```python
from build123d import *

# Parameters (mm, degrees)
PAD_DEPTH       = 15
FILLET_R        = 10
FILLET001_R     = 3
CHAMFER_SIZE    = 2
FILLET002_R     = 0.5
FILLET003_R     = 5
CHAMFER001_SIZE = 0.25
SKETCH003_R     = 1.5
POCKET_DEPTH    = 33.001


with BuildPart() as sweep_body:
    # Sweep: sweep along a path in Sketch001
    with BuildLine(Plane.XY) as sweep_path:
        Line((21, -10), (21, 15.000008))
        ThreePointArc((21, 15.000008), (18.071065, 22.071071), (11, 25))
        Line((11, 25), (-11, 25))
        ThreePointArc((-11, 25), (-18.071068, 22.071068), (-21, 15))
        Line((-21, 15), (-21, -10))
    # Sketch002 → Sweep (sweep)
    with BuildSketch(Plane.XZ.offset(10)):
        Polygon((22, 3.25), (22, -3.25), (20, -1.25), (20, 1.25), align=None)
    sweep(path=sweep_path.line)


with BuildPart() as sweep_body_1:
    # Sweep placement: moved
    add(sweep_body.part.moved(Location((0, 0, 3))))


with BuildPart() as fusion:
    # Clone base: copy of Sweep body
    add(sweep_body_1.part)


with BuildPart() as fusion_1:
    # Clone placement: moved
    add(fusion.part.moved(Location((0, 0, 9))))

    # Fusion: union Sweep body
    add(sweep_body_1.part)


with BuildPart() as pocket:
    # Sketch → Pad (new body)
    with BuildSketch(Plane.XY):
        Polygon((-18, -8), (-18, 12), (-12, 18), (12, 18), (18, 12), (18, -8), (21, -8), (21, 25), (-21, 25), (-21, -8), align=None)
    extrude(amount=PAD_DEPTH)

    # Fillet
    fillet_edges = [pocket.edges().sort_by_distance(p)[0] for p in [
        (-21, 25, 7.5),
        (21, 25, 7.5),
    ]]
    fillet(fillet_edges, radius=FILLET_R)

    # Fillet001
    fillet001_edges = [pocket.edges().sort_by_distance(p)[0] for p in [
        (-12, 18, 7.5),
        (-18, 12, 7.5),
        (12, 18, 7.5),
        (18, 12, 7.5),
    ]]
    fillet(fillet001_edges, radius=FILLET001_R)

    # Chamfer
    chamfer_edges = [pocket.edges().sort_by_distance(p)[0] for p in [
        (-21, -8, 7.5),
        (21, -8, 7.5),
    ]]
    chamfer(chamfer_edges, length=CHAMFER_SIZE)

    # Fillet002
    fillet002_edges = [pocket.edges().sort_by_distance(p)[0] for p in [
        (-19, -8, 7.5),
        (-18, -8, 7.5),
        (19, -8, 7.5),
        (18, -8, 7.5),
    ]]
    fillet(fillet002_edges, radius=FILLET002_R)

    # Fillet003
    fillet003_edges = [pocket.edges().sort_by_distance(p)[0] for p in [
        (-21, -6, 7.5),
        (21, -6, 7.5),
    ]]
    fillet(fillet003_edges, radius=FILLET003_R)

    # Chamfer001
    chamfer001_edges = [pocket.edges().sort_by_distance(p)[0] for p in [
        (19.34099, -7.65901, 15),
        (20.619398, -5.842349, 15),
        (18.984235, -7.96194, 15),
        (21, 5.535534, 15),
        (18.646447, -8, 15),
        (18.071068, 22.071068, 15),
        (18.146447, -7.853553, 15),
        (0, 25, 15),
        (18, 1.62868, 15),
        (-18.071068, 22.071068, 15),
        (17.771639, 11.90541, 15),
        (-21, 5.535534, 15),
        (15, 15, 15),
        (-20.619398, -5.842349, 15),
        (11.90541, 17.771639, 15),
        (-19.34099, -7.65901, 15),
        (0, 18, 15),
        (-18.984235, -7.96194, 15),
        (-11.90541, 17.771639, 15),
        (-18.646447, -8, 15),
        (-15, 15, 15),
        (-18.146447, -7.853553, 15),
        (-17.771639, 11.90541, 15),
        (-18, 1.62868, 15),
        (19.34099, -7.65901, 0),
        (20.619398, -5.842349, 0),
        (18.984235, -7.96194, 0),
        (21, 5.535534, 0),
        (18.646447, -8, 0),
        (18.071068, 22.071068, 0),
        (18.146447, -7.853553, 0),
        (0, 25, 0),
        (18, 1.62868, 0),
        (-18.071068, 22.071068, 0),
        (17.771639, 11.90541, 0),
        (-21, 5.535534, 0),
        (15, 15, 0),
        (-20.619398, -5.842349, 0),
        (11.90541, 17.771639, 0),
        (-19.34099, -7.65901, 0),
        (0, 18, 0),
        (-18.984235, -7.96194, 0),
        (-11.90541, 17.771639, 0),
        (-18.646447, -8, 0),
        (-15, 15, 0),
        (-18.146447, -7.853553, 0),
        (-17.771639, 11.90541, 0),
        (-18, 1.62868, 0),
    ]]
    chamfer(chamfer001_edges, length=CHAMFER001_SIZE)

    # Cut: cut Fusion
    add(fusion_1.part, mode=Mode.SUBTRACT)

    # Sketch003 → Pocket (cut, through all)
    with BuildSketch(Plane(origin=(0, 25, 0), x_dir=(-1, 0, 0), z_dir=(0, 1, 0))):
        with Locations((-12, 7.5)):
            Circle(SKETCH003_R)
        with Locations((0, 7.5)):
            Circle(SKETCH003_R)
        with Locations((12, 7.5)):
            Circle(SKETCH003_R)
    extrude(amount=-POCKET_DEPTH, mode=Mode.SUBTRACT)


solid = pocket.part
```
Check sheet for the modelled part. Datum: model origin and axes. Units: mm. A direction names the side the tool comes from. Give positions to 0.01 mm unless a question says otherwise; leave off trailing zeros. Write each loop counter-clockwise with the first axis right and the second up, starting at its lowest first coordinate (ties: lowest second). Pieces come first, ordered by that corner, then holes. Notation, with made-up numbers: (32, 88) - (40, 88) arc R23 cw to (40, 120) - close; hole circle Ø8 at (35, 18.25). An arc over 180 degrees is marked (long way). Answer as a JSON object with one key per item and string values. Group by question number.
1) Release check for a two-part mould opening along Z. For faces 1 (the face through (17.78, 11.89, 7.6)), 2 (the face through (0, 24, 12)), 3 (the face through (-17.91, 22.06, 0.13)), 4 (the face through (13.5, 21.72, 7.57)) record: pulls with the +Z half, pulls with the -Z half, needs draft (parallel to the pull), parting line crosses it, or undercut.
2) Depth check by flat-ended pin: P1, Ø1.3, axis at y = 4.5, z = 11.5, coming from the -X side; P2, Ø1.2, axis at y = 6, z = 12.5, coming from the +X side; P3, Ø3, axis at y = 6, z = 3, coming from the -X side. Enter the tip coordinate at first touch or a pass-through.
3) Access from +Z, -Z, +X, -X, +Y, -Y to the whole of each face (thin tool, end or side, straight path). Record for faces 5 (the face through (11.921, 17.765, 3.5)), 6 (the face through (20.49, 4.19, 10.26)), 7 (the face through (11.94, 17.89, 0.13)).
4) Sectioned sample at B-B (x = 0). Record the cut outline in (y, z), then the cut area to 3 significant figures.
5) Sectioned sample at C-C (z = 7.5). Give the number of separate pieces and of enclosed holes in the cut face, then the cut area to 3 significant figures.
6) Sectioned sample at D-D (z = 12.5). Record the cut outline in (x, y).
7) Thickness scan on probe 1 along Z at (x, y) = (-12, 23); probe 2 along X at (y, z) = (-3.5, 12.5); probe 3 along Y at (x, z) = (8.5, 7.5). Record the ranges inside material, lowest first. Write a range as from..to.
Geometry results:
{
 "1": {"face 1": "needs draft", "face 2": "undercut", "face 3": "pulls with the -Z half", "face 4": "undercut"},
 "2": {"P1": "stops at x = -20", "P2": "stops at x = 20", "P3": "stops at x = -20.25"},
 "3": {"face 5": "+Z, -Z, -Y", "face 6": "+X, +Y, -Y", "face 7": "-Z, -Y"},
 "4": {"outline": "(18, 0.25) - (18.25, 0) - (24.75, 0) - (25, 0.25) - (25, 0.75) - (24, 1.75) - (24, 4.25) - (25, 5.25) - (25, 6) - (18, 6) - close; (18, 9) - (25, 9) - (25, 9.75) - (24, 10.75) - (24, 13.25) - (25, 14.25) - (25, 14.75) - (24.75, 15) - (18.25, 15) - (18, 14.75) - close", "area": "76.9 mm^2"},
 "5": {"separate pieces": "4", "enclosed holes": "0", "area": "374 mm^2"},
 "6": {"outline": "(-20, -6.93) arc R5 ccw to (-19.54, -7.46) - (-19.15, -7.85) arc R0.5 ccw to (-18.79, -8) - (-18.5, -8) arc R0.5 ccw to (-18, -7.5) - (-18, 10.76) arc R3 cw to (-17.12, 12.88) - (-12.88, 17.12) arc R3 cw to (-10.76, 18) - (10.76, 18) arc R3 cw to (12.88, 17.12) - (17.12, 12.88) arc R3 cw to (18, 10.76) - (18, -7.5) arc R0.5 ccw to (18.5, -8) - (18.79, -8) arc R0.5 ccw to (19.15, -7.85) - (19.54, -7.46) arc R5 ccw to (20, -6.93) - (20, 15) arc R9 ccw to (11, 24) - (-11, 24) arc R9 ccw to (-20, 15) - close"},
 "7": {"probe 1": "z = 0..6, 9..15", "probe 2": "x = -20..-18, 18..20", "probe 3": "y = 18..25"}
}
